Source: CAD feature listing. Evaluate the final solid. Frame: model axes, mm. Coordinates: 2 decimals unless noted, no trailing zeros. Loops run counter-clockwise (first coordinate to the right, second up) from the corner with the lowest first, then second, coordinate; pieces in that order, holes last.
```python
from build123d import *

# Parameters (mm, degrees)
CYLINDER071_R     = 1.3
CYLINDER071_DEPTH = 331
CYLINDER062_R     = 1.3
CYLINDER062_DEPTH = 331
CYLINDER052_W     = 105
CYLINDER052_H     = 10
CYLINDER052_ANGLE = 180
CYLINDER051_W     = 115
CYLINDER051_H     = 10
CYLINDER051_ANGLE = 180


with BuildPart() as cilindro071:
    # Cylinder071 → Cylinder071 (new body)
    with BuildSketch(Plane(origin=(5, 224, 178), x_dir=(0, 0, -1), z_dir=(1, 0, 0))):
        Circle(CYLINDER071_R)
    extrude(amount=CYLINDER071_DEPTH)


with BuildPart() as cilindro062:
    # Cylinder062 → Cylinder062 (new body)
    with BuildSketch(Plane(origin=(5, 6, 178), x_dir=(0, 0, -1), z_dir=(1, 0, 0))):
        Circle(CYLINDER062_R)
    extrude(amount=CYLINDER062_DEPTH)


with BuildPart() as cilindro052:
    # Cylinder052 → Cylinder052 (revolve)
    with BuildSketch(Plane(origin=(-3, 115, 171), x_dir=(0, -1, 0), z_dir=(0, 0, -1))):
        with Locations((52.5, 5)):
            Rectangle(CYLINDER052_W, CYLINDER052_H)
    revolve(axis=Axis((-3, 115, 171), (-1, 0, 0)), revolution_arc=CYLINDER052_ANGLE)


with BuildPart() as cut080:
    # Cylinder051 → Cylinder051 (revolve)
    with BuildSketch(Plane(origin=(-3, 115, 171), x_dir=(0, -1, 0), z_dir=(0, 0, -1))):
        with Locations((57.5, 5)):
            Rectangle(CYLINDER051_W, CYLINDER051_H)
    revolve(axis=Axis((-3, 115, 171), (-1, 0, 0)), revolution_arc=CYLINDER051_ANGLE)

    # Cut066: cut Cilindro052
    add(cilindro052.part, mode=Mode.SUBTRACT)


with BuildPart() as cut080_1:
    # Cut066 placement: moved
    add(cut080.part.moved(Location((13, 0, -9))))

    # Cut073: cut Cilindro062
    add(cilindro062.part, mode=Mode.SUBTRACT)

    # Cut080: cut Cilindro071
    add(cilindro071.part, mode=Mode.SUBTRACT)


solid = cut080_1.part
```
Q1. Section query A-A on z = 200. Return the cut outline in (x, y), then the cut area to 3 significant figures.
Q2. Section query C-C on z = 241. Return the cut outline in (x, y), then the cut area to 3 significant figures.
Q3. Section query B-B on x = 6.75. Return the cut outline in (y, z).
Q4. Draft query along Y for faces 1 (the cylindrical face through (4.93, 112.691, 266.975)), 2 (the cylindrical face through (4.93, 112.471, 276.972)), 3 (the flat face through (5, 5, 162)). Return one class per face: released by +Y, released by -Y, zero draft, split by the parting line, or undercut.
Q5. Section query D-D on y = 212. Return the cut outline in (x, z).
Q6. First-contact query: pin 1 Ø3 at (x, y) = (1.5, 59.5) entering from +Z; pin 2 Ø0.8 at (y, z) = (6, 177.5) entering from +X; pin 3 Ø4 at (y, z) = (191, 252.5) entering from -X; pin 4 Ø5 at (x, y) = (2.5, 119.5) entering from -Z. Flat tips, straight axial feed; report the tip coordinate or a pass-through.
Q7. Material intervals for line 1 along Y through (x, z) = (7.85, 178); line 2 along Y through (x, z) = (7, 231); line 3 along Y through (x, z) = (7.5, 172.5), sorted ascending.
Resolved:
1. outline: (0, 6.46) - (10, 6.46) - (10, 17.12) - (0, 17.12) - close; (0, 212.88) - (10, 212.88) - (10, 223.54) - (0, 223.54) - close
1. area: 213 mm2
2. outline: (0, 31.43) - (10, 31.43) - (10, 45.83) - (0, 45.83) - close; (0, 184.17) - (10, 184.17) - (10, 198.57) - (0, 198.57) - close
2. area: 288 mm2
3. outline: (0, 162) - (10, 162) arc R105 cw to (220, 162) - (230, 162) arc R115 ccw to start; hole circle Ø2.6 at (6, 178); hole circle Ø2.6 at (224, 178)
4. face 1: undercut
4. face 2: split by the parting line
4. face 3: zero draft
5. outline: (0, 202.2) - (10, 202.2) - (10, 223.77) - (0, 223.77) - close
6. pin 1: stops at z = 263.53
6. pin 2: stops at x = 5
6. pin 3: passes through
6. pin 4: stops at z = 266.77
7. line 1: y = 1.12 to 4.7, 7.3 to 11.23, 218.77 to 222.7, 225.3 to 228.88
7. line 2: y = 23 to 35.85, 194.15 to 207
7. line 3: y = 0.48 to 10.53, 219.47 to 229.52
